Could you check a few things on this model? Use its own coordinates, in mm. Round coordinates to 2 decimals unless told otherwise and drop trailing zeros. Order: outer loops, then holes, each group sorted by start corner. A loop starts at its lowest first (then second) coordinate and runs counter-clockwise, first axis right, second up. Notation, with made-up numbers: (83, 42.25) -> (101, 42.25) arc R12 cw to (101, 59.25) -> close; hole circle Ø6 at (13.5, 50.5). An arc over 180 degrees is marked (long way). One line per question, with ' | ' between items.
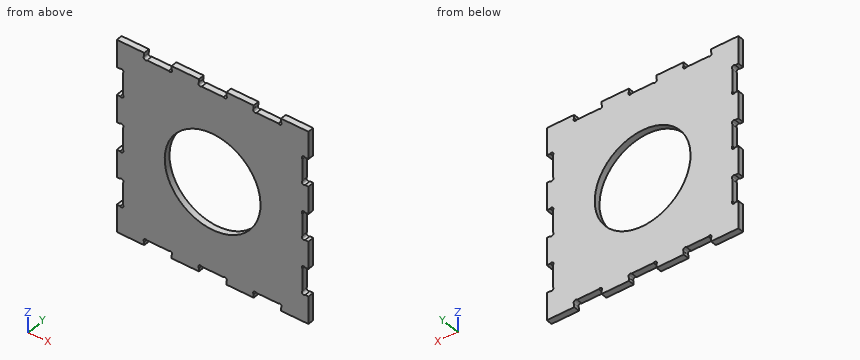
```python
from build123d import *

# Parameters (mm, degrees)
SKETCH1_W                   = 100
SKETCH1_H                   = 100
BOSS_EXTRUDE1_DEPTH         = 3.18
SKETCH2_W                   = 14.285714285
SKETCH2_H                   = 3.18
SKETCH2_W_2                 = 14.285714286
CUT_EXTRUDE1_DEPTH          = 71.782147467
SKETCH3_R                   = 1
CUT_EXTRUDE2_DEPTH          = 71.782147467
SKETCH_PATTERN1_DEPTH       = 3.18
CIRPATTERN1_COUNT           = 4
CIRPATTERN1_COPY_1_SKETCH_R = 1
CIRPATTERN1_COPY_1_DEPTH    = 71.782147467
CIRPATTERN1_COPY_2_SKETCH_R = 1
CIRPATTERN1_COPY_2_DEPTH    = 71.782147467
CIRPATTERN1_COPY_3_SKETCH_R = 1
CIRPATTERN1_COPY_3_DEPTH    = 71.782147467
CIRPATTERN1_COPY_4_DEPTH    = 3.18
CIRPATTERN1_COPY_5_DEPTH    = 3.18
CIRPATTERN1_COPY_6_DEPTH    = 3.18
CUT_EXTRUDE3_DEPTH          = 71.782147467
CUT_EXTRUDE3_DEPTH_BACK     = 71.782147467
SKETCH5_R                   = 25


# Read off the part's stored shape, not the designer's step: Sketch-Pattern1
with BuildPart() as part:
    # Sketch1 → Boss-Extrude1 (new body)
    with BuildSketch(Plane(origin=(0, 0, 0), x_dir=(1, 0, 0), z_dir=(0, 1, 0))):
        Rectangle(SKETCH1_W, SKETCH1_H)
    extrude(amount=BOSS_EXTRUDE1_DEPTH)

    # Sketch2 → Cut-Extrude1 (cut, symmetric)
    with BuildSketch(Plane(origin=(0, 3.18, 0), x_dir=(1, 0, 0), z_dir=(0, 1, 0))):
        with Locations((-28.571428572, 48.41)):
            Rectangle(SKETCH2_W, SKETCH2_H)
        with Locations((0, 48.41)):
            Rectangle(SKETCH2_W_2, SKETCH2_H)
        with Locations((28.571428572, 48.41)):
            Rectangle(SKETCH2_W, SKETCH2_H)
    cut_extrude1 = extrude(amount=CUT_EXTRUDE1_DEPTH, both=True, mode=Mode.SUBTRACT)

    # Sketch3 → Cut-Extrude2 (cut, symmetric)
    with BuildSketch(Plane(origin=(0, 3.18, 0), x_dir=(1, 0, 0), z_dir=(0, 1, 0))):
        with Locations((-35.007178933, 47.527106781)):
            Circle(SKETCH3_R)
    cut_extrude2 = extrude(amount=CUT_EXTRUDE2_DEPTH, both=True, mode=Mode.SUBTRACT)

    # Sketch-Pattern1 outline → Sketch-Pattern1 (cut)
    with BuildSketch(Plane(origin=(0, 0, 0), x_dir=(1, 0, 0), z_dir=(0, 1, 0))):
        with BuildLine():
            Line((-7.142857143, 46.82), (-7.142857143, 48.234213562))
            ThreePointArc((-7.142857143, 48.234213562), (-7.435750362, 47.527106781), (-7.142857143, 46.82))
        make_face()
        with BuildLine():
            Line((-5.72864358, 46.82), (-7.142857143, 46.82))
            ThreePointArc((-7.142857143, 46.82), (-6.435750362, 46.527106781), (-5.72864358, 46.82))
        make_face()
        with BuildLine():
            Line((21.428571429, 46.82), (21.428571429, 48.234213562))
            ThreePointArc((21.428571429, 48.234213562), (21.13567821, 47.527106781), (21.428571429, 46.82))
        make_face()
        with BuildLine():
            Line((22.842784991, 46.82), (21.428571429, 46.82))
            ThreePointArc((21.428571429, 46.82), (22.13567821, 46.527106781), (22.842784991, 46.82))
        make_face()
    sketch_pattern1 = extrude(amount=SKETCH_PATTERN1_DEPTH, mode=Mode.SUBTRACT)

    # Mirror1: Cut-Extrude2, Sketch-Pattern1 across plane
    add(cut_extrude2.mirror(Plane(origin=(0, 0, 0), x_dir=(0, 0, 1), z_dir=(1, 0, 0))), mode=Mode.SUBTRACT)
    add(sketch_pattern1.mirror(Plane(origin=(0, 0, 0), x_dir=(0, 0, 1), z_dir=(1, 0, 0))), mode=Mode.SUBTRACT)

    # CirPattern1: Cut-Extrude1, Cut-Extrude2, Sketch-Pattern1 ×4 about axis
    cirpattern1_axis = Axis((0, 0, 0), (0, 1, 0))
    add([cut_extrude1.rotate(cirpattern1_axis, i * 360 / CIRPATTERN1_COUNT) for i in range(1, CIRPATTERN1_COUNT)], mode=Mode.SUBTRACT)
    add([cut_extrude2.rotate(cirpattern1_axis, i * 360 / CIRPATTERN1_COUNT) for i in range(1, CIRPATTERN1_COUNT)], mode=Mode.SUBTRACT)
    add([sketch_pattern1.rotate(cirpattern1_axis, i * 360 / CIRPATTERN1_COUNT) for i in range(1, CIRPATTERN1_COUNT)], mode=Mode.SUBTRACT)

    # CirPattern1 copy 1 sketch → CirPattern1 copy 1 (cut, symmetric)
    with BuildSketch(Plane.ZX.offset(3.18)):
        with Locations((-35.007178933, -47.527106781)):
            Circle(CIRPATTERN1_COPY_1_SKETCH_R)
    extrude(amount=CIRPATTERN1_COPY_1_DEPTH, both=True, mode=Mode.SUBTRACT)

    # CirPattern1 copy 2 sketch → CirPattern1 copy 2 (cut, symmetric)
    with BuildSketch(Plane(origin=(0, 3.18, 0), x_dir=(1, 0, 0), z_dir=(0, 1, 0))):
        with Locations((-35.007178933, -47.527106781)):
            Circle(CIRPATTERN1_COPY_2_SKETCH_R)
    extrude(amount=CIRPATTERN1_COPY_2_DEPTH, both=True, mode=Mode.SUBTRACT)

    # CirPattern1 copy 3 sketch → CirPattern1 copy 3 (cut, symmetric)
    with BuildSketch(Plane(origin=(0, 3.18, 0), x_dir=(0, 0, -1), z_dir=(0, 1, 0))):
        with Locations((-35.007178933, -47.527106781)):
            Circle(CIRPATTERN1_COPY_3_SKETCH_R)
    extrude(amount=CIRPATTERN1_COPY_3_DEPTH, both=True, mode=Mode.SUBTRACT)

    # CirPattern1 copy 4 sketch → CirPattern1 copy 4 (cut)
    with BuildSketch(Plane.ZX):
        with BuildLine():
            Line((-7.142857143, -46.82), (-7.142857143, -48.234213562))
            ThreePointArc((-7.142857143, -48.234213562), (-7.435750362, -47.527106781), (-7.142857143, -46.82))
        make_face()
        with BuildLine():
            Line((-5.72864358, -46.82), (-7.142857143, -46.82))
            ThreePointArc((-7.142857143, -46.82), (-6.435750362, -46.527106781), (-5.72864358, -46.82))
        make_face()
        with BuildLine():
            Line((21.428571429, -46.82), (21.428571429, -48.234213562))
            ThreePointArc((21.428571429, -48.234213562), (21.13567821, -47.527106781), (21.428571429, -46.82))
        make_face()
        with BuildLine():
            Line((22.842784991, -46.82), (21.428571429, -46.82))
            ThreePointArc((21.428571429, -46.82), (22.13567821, -46.527106781), (22.842784991, -46.82))
        make_face()
    extrude(amount=CIRPATTERN1_COPY_4_DEPTH, mode=Mode.SUBTRACT)

    # CirPattern1 copy 5 sketch → CirPattern1 copy 5 (cut)
    with BuildSketch(Plane(origin=(0, 0, 0), x_dir=(1, 0, 0), z_dir=(0, 1, 0))):
        with BuildLine():
            Line((-7.142857143, -46.82), (-7.142857143, -48.234213562))
            ThreePointArc((-7.142857143, -48.234213562), (-7.435750362, -47.527106781), (-7.142857143, -46.82))
        make_face()
        with BuildLine():
            Line((-5.72864358, -46.82), (-7.142857143, -46.82))
            ThreePointArc((-7.142857143, -46.82), (-6.435750362, -46.527106781), (-5.72864358, -46.82))
        make_face()
        with BuildLine():
            Line((21.428571429, -46.82), (21.428571429, -48.234213562))
            ThreePointArc((21.428571429, -48.234213562), (21.13567821, -47.527106781), (21.428571429, -46.82))
        make_face()
        with BuildLine():
            Line((22.842784991, -46.82), (21.428571429, -46.82))
            ThreePointArc((21.428571429, -46.82), (22.13567821, -46.527106781), (22.842784991, -46.82))
        make_face()
    extrude(amount=CIRPATTERN1_COPY_5_DEPTH, mode=Mode.SUBTRACT)

    # CirPattern1 copy 6 sketch → CirPattern1 copy 6 (cut)
    with BuildSketch(Plane(origin=(0, 0, 0), x_dir=(0, 0, -1), z_dir=(0, 1, 0))):
        with BuildLine():
            Line((-7.142857143, -46.82), (-7.142857143, -48.234213562))
            ThreePointArc((-7.142857143, -48.234213562), (-7.435750362, -47.527106781), (-7.142857143, -46.82))
        make_face()
        with BuildLine():
            Line((-5.72864358, -46.82), (-7.142857143, -46.82))
            ThreePointArc((-7.142857143, -46.82), (-6.435750362, -46.527106781), (-5.72864358, -46.82))
        make_face()
        with BuildLine():
            Line((21.428571429, -46.82), (21.428571429, -48.234213562))
            ThreePointArc((21.428571429, -48.234213562), (21.13567821, -47.527106781), (21.428571429, -46.82))
        make_face()
        with BuildLine():
            Line((22.842784991, -46.82), (21.428571429, -46.82))
            ThreePointArc((21.428571429, -46.82), (22.13567821, -46.527106781), (22.842784991, -46.82))
        make_face()
    extrude(amount=CIRPATTERN1_COPY_6_DEPTH, mode=Mode.SUBTRACT)

    # Sketch5 → Cut-Extrude3 (cut, two sides: drawn at the far end of the back side and taken through both)
    with BuildSketch(Plane(origin=(0, 3.18, 0), x_dir=(1, 0, 0), z_dir=(0, 1, 0)).offset(-CUT_EXTRUDE3_DEPTH_BACK)):
        with Locations(Location((0, 0, 0), (0, 0, 270))):
            Circle(SKETCH5_R)
    extrude(amount=CUT_EXTRUDE3_DEPTH + CUT_EXTRUDE3_DEPTH_BACK, mode=Mode.SUBTRACT)


solid = part.part
```
1. I want a section at C-C on x = 32.5. List the corners of the cut face in (y, z) for me, and give its area (3 significant figures).
From the geometry:
outline: (0, -46.82) -> (3.18, -46.82) -> (3.18, 46.82) -> (0, 46.82) -> close | area: 298 mm²
2. I need wall thicknesses on probe 1 along X at (y, z) = (1.9, 0); probe 2 along Z at (x, y) = (-35, 0.75). Which ranges of each line are inside material? Lowest first, please.
From the geometry:
probe 1: x = -46.82 to -25, 25 to 46.82 | probe 2: z = -46.53 to 46.53
3. I want a section at B-B on z = 0. List the corners of the cut face in (x, y) for me, and give its area (3 significant figures).
From the geometry:
outline: (-46.82, 0) -> (-25, 0) -> (-25, 3.18) -> (-46.82, 3.18) -> close; (25, 0) -> (46.82, 0) -> (46.82, 3.18) -> (25, 3.18) -> close | area: 139 mm²
4. I want a section at D-D on z = -32.5. List the corners of the cut face in (x, y) for me.
From the geometry:
outline: (-46.82, 0) -> (46.82, 0) -> (46.82, 3.18) -> (-46.82, 3.18) -> close
5. I want a section at A-A on x = 0. List the corners of the cut face in (y, z) for me, and give its area (3 significant figures).
From the geometry:
outline: (0, -46.82) -> (3.18, -46.82) -> (3.18, -25) -> (0, -25) -> close; (0, 25) -> (3.18, 25) -> (3.18, 46.82) -> (0, 46.82) -> close | area: 139 mm²
6. I'm going to push flat-ended pins straight in: pin 1 (1 mm diameter, centred on y = 1.5, z = 32.5, fed in from +X); pin 2 (1 mm diameter, centred on x = 28, y = 1.5, fed in from -Z); pin 3 (1.6 mm diameter, centred on x = -27.5, y = 2.5, fed in from +Z). Where does each tip first touch, or does it pass through?
From the geometry:
pin 1: stops at x = 46.82 | pin 2: stops at z = -46.82 | pin 3: stops at z = 46.82
